Solid Edge part; units mm, degrees
sketch "Sketch1" plane through (0, 0, 0) normal (1, 0, 0) x (0, 1, 0)
  line L0 (-57.7882, -59) -> (60.2118, -59)
  line L1 (60.2118, -59) -> (60.2118, 59)
  line L2 (60.2118, 59) -> (-57.7882, 59)
  line L3 (-57.7882, 59) -> (-57.7882, -59)
extrude "Protrusion1" add sketch "Sketch1" against normal blind 22
sketch "Sketch2" plane through (0, 1.2118, 0) normal (1, 0, 0) x (0, 1, 0)
  line L0 (-37, 33) -> (-37, -33)
  line L1 (-37, -33) -> (-11, -33)
  line L2 (-11, -33) -> (-11, 33)
  line L3 (-37, 33) -> (-11, 33)
extrude "ExtrudedCutout_1" cut sketch "Sketch2" against normal blind 50
sketch "Sketch3" plane through (0, 1.2118, 0) normal (1, 0, 0) x (0, 1, 0)
  line L0 (37, 33) -> (37, -33)
  line L1 (11, -33) -> (37, -33)
  line L2 (11, -33) -> (11, 33)
  line L3 (11, 33) -> (37, 33)
extrude "ExtrudedCutout_2" cut sketch "Sketch3" against normal blind 28
sketch "Sketch4" plane through (-11, -57.7882, 0) normal (0, -1, 0) x (0, 0, -1)
  line L0 (-59, 11) -> (59, 11)
  line L1 (-59, 11) -> (-59, 6.4)
  line L2 (-59, 6.4) -> (59, 6.4)
  line L3 (59, 6.4) -> (59, 11)
extrude "ExtrudedCutout_3" cut sketch "Sketch4" against normal blind 5
sketch "Sketch5" plane through (-13.3, -57.7882, 0) normal (0, -1, 0) x (0, 0, -1)
  line L0 (-59, -4.1) -> (59, -4.1)
  line L1 (59, -4.1) -> (59, -8.7)
  line L2 (59, -8.7) -> (-59, -8.7)
  line L3 (-59, -8.7) -> (-59, -4.1)
extrude "ExtrudedCutout_4" cut sketch "Sketch5" against normal blind 5
sketch "Sketch6" plane through (0, 3.7118, 0) normal (1, 0, 0) x (0, 1, 0)
  line L0 (-39.5, -37) -> (-39.5, -59)
  line L1 (-39.5, -59) -> (-44.5, -59)
  line L2 (-44.5, -59) -> (-44.5, 59)
  line L3 (-44.5, 59) -> (-39.5, 59)
  line L4 (-39.5, 59) -> (-39.5, -37)
extrude "ExtrudedCutout_5" cut sketch "Sketch6" against normal blind 4.6
sketch "Sketch7" plane through (-11, 1.2118, -59) normal (0, 0, -1) x (0, 1, 0)
  line L0 (-42, -11) -> (-42, -6.4)
  line L1 (-42, -6.4) -> (-37, -6.4)
  line L2 (-37, -6.4) -> (-37, -11)
  line L3 (-37, -11) -> (-42, -11)
extrude "ExtrudedCutout_6" cut sketch "Sketch7" against normal blind 120
sketch "Sketch8" plane through (0, 12.2118, 0) normal (1, 0, 0) x (0, 1, 0)
  line L0 (-22, -33) -> (-22, -59)
  line L1 (-22, -59) -> (-17, -59)
  line L2 (-17, -59) -> (-17, 59)
  line L3 (-17, 59) -> (-22, 59)
  line L4 (-22, 59) -> (-22, -33)
extrude "ExtrudedCutout_7" cut sketch "Sketch8" against normal blind 4.6
sketch "Sketch9" plane through (0, 27.7118, 0) normal (1, 0, 0) x (0, 1, 0)
  line L0 (-15.5, -33) -> (-15.5, -59)
  line L1 (-15.5, -59) -> (-20.5, -59)
  line L2 (-20.5, -59) -> (-20.5, 59)
  line L3 (-20.5, 59) -> (-15.5, 59)
  line L4 (-15.5, 59) -> (-15.5, -33)
extrude "ExtrudedCutout_8" cut sketch "Sketch9" against normal blind 4.6
sketch "Sketch10" plane through (-11, 1.2118, 59) normal (0, 0, 1) x (0, 1, 0)
  line L0 (-6, 11) -> (-6, 6.4)
  line L1 (-6, 6.4) -> (-11, 6.4)
  line L2 (-11, 6.4) -> (-11, 11)
  line L3 (-11, 11) -> (-6, 11)
  line L4 (11, 6.4) -> (6, 6.4)
  line L5 (6, 6.4) -> (6, 11)
  line L6 (6, 11) -> (11, 11)
  line L7 (11, 11) -> (11, 6.4)
extrude "Cutout1" cut sketch "Sketch10" against normal blind 118
sketch "Sketch11" plane through (0, 36.2118, 0) normal (1, 0, 0) x (0, 1, 0)
  line L0 (2, -59) -> (7, -59)
  line L1 (7, -59) -> (7, 59)
  line L2 (7, 59) -> (2, 59)
  line L3 (2, 59) -> (2, -59)
extrude "ExtrudedCutout_10" cut sketch "Sketch11" against normal blind 4.6
sketch "Sketch12" plane through (0, 51.7118, 0) normal (1, 0, 0) x (0, 0, -1)
  line L0 (59, 8.5) -> (59, 3.5)
  line L1 (59, 3.5) -> (-59, 3.5)
  line L2 (-59, 3.5) -> (-59, 8.5)
  line L3 (-59, 8.5) -> (59, 8.5)
extrude "ExtrudedCutout_11" cut sketch "Sketch12" against normal blind 4.6
sketch "Sketch13" plane through (-11, 1.2118, 59) normal (0, 0, 1) x (0, 1, 0)
  line L0 (42, 11) -> (42, 6.4)
  line L1 (42, 6.4) -> (37, 6.4)
  line L2 (37, 11) -> (37, 6.4)
  line L3 (42, 11) -> (37, 11)
  line L4 (54, 6.4) -> (59, 6.4)
  line L5 (59, 6.4) -> (59, 11)
  line L6 (59, 11) -> (54, 11)
  line L7 (54, 11) -> (54, 6.4)
extrude "ExtrudedCutout_12" cut sketch "Sketch13" against normal blind 118
properties material "Stainless steel"
Model file for the job. Use its own axes, mm. A direction names the side the tool comes from. Coordinates: 2 decimals unless noted, no trailing zeros. Order: outer loops, then holes, each group sorted by start corner. A loop starts at its lowest first (then second) coordinate and runs counter-clockwise, first axis right, second up. Notation, with made-up numbers: (-30.75, 29) -> (-24.75, 29) arc R19 ccw to (-24.75, 44) -> close; hole circle Ø7 at (-35.5, -17). An arc over 180 degrees is marked (long way). Answer as a JSON object with one key per item and string values. Group by question number.
1) Which spindle directions (+Z, -Z, +X, -X, +Y, -Y) get a long thin tool onto all of the face, cutting with end or side? Do faces 1 (the face through (-4.6, -38, 1)), 2 (the face through (-11, -9.788, 0)), 3 (the face through (-20, 55.212, 1)), 4 (the face through (-20, -35.788, 46)), 5 (the face through (-4.6, 58, 1)). Say none if no direction does.
2) Flat gauge pins, fed straight in: pin 1 (1.4 mm diameter, centred on x = -20, z = 19.5, fed in from -Y); pin 2 (2 mm diameter, centred on y = 41.5, z = -39, fed in from -X); pin 3 (5.5 mm diameter, centred on y = 58.5, z = -1, fed in from +X). Where does each tip first touch, or does it go through?
3) Cut at C-C, the plane z = -9. Count the separate pieces of the cut face and the enclosed holes in it, then the cut area to 3 significant figures.
4) Drill centre lines: L1, parallel to Y at x = -4.25, z = 42; L2, parallel to Y at x = -17, z = 12; L3, parallel to Y at x = -3.5, z = -30. Where is each one in solid material? Low to high.
5) Cut at A-A, the plane x = -19. Write the cut outline in (y, z), then the cut area to 3 significant figures.
6) Cut at B-B, the plane y = 28. Write the cut outline in (x, z), then the cut area to 3 significant figures.
Check values:
{
 "1": {"face 1": "+Z, -Z, +X", "face 2": "+X, -X", "face 3": "+Z, -Z, -X, +Y", "face 4": "+Z, -Z, -X", "face 5": "+Z, -Z, +X, +Y"},
 "2": {"pin 1": "stops at y = -52.79", "pin 2": "stops at x = -17.4", "pin 3": "stops at x = -4.6"},
 "3": {"separate pieces": "3", "enclosed holes": "0", "area": "1,180 mm²"},
 "4": {"L1": "y = -52.79 to -40.79, -35.79 to -9.79, -4.79 to 7.21, 12.21 to 38.21, 43.21 to 55.21", "L2": "y = -57.79 to -35.79, -9.79 to 12.21, 38.21 to 60.21", "L3": "y = -52.79 to -40.79, -4.79 to 7.21, 43.21 to 55.21"},
 "5": {"outline": "(-52.79, -59) -> (-40.79, -59) -> (-40.79, 59) -> (-52.79, 59) -> close; (-35.79, -59) -> (-9.79, -59) -> (-9.79, -33) -> (-35.79, -33) -> close; (-35.79, 33) -> (-9.79, 33) -> (-9.79, 59) -> (-35.79, 59) -> close; (-4.79, -59) -> (7.21, -59) -> (7.21, 59) -> (-4.79, 59) -> close; (12.21, -59) -> (38.21, -59) -> (38.21, -33) -> (12.21, -33) -> close; (12.21, 33) -> (38.21, 33) -> (38.21, 59) -> (12.21, 59) -> close; (43.21, -59) -> (55.21, -59) -> (55.21, 59) -> (43.21, 59) -> close", "area": "6,950 mm²"},
 "6": {"outline": "(-22, -59) -> (0, -59) -> (0, -33) -> (-22, -33) -> close; (-22, 33) -> (0, 33) -> (0, 59) -> (-22, 59) -> close", "area": "1,140 mm²"}
}
